Autodesk Inventor part; units mm, degrees
ref_plane "Start plane" through (0, 0, 25) normal (0, 0, 1) x (1, 0, 0)
ref_plane "End plane" through (0, 0, 285) normal (0, 0, 1) x (1, 0, 0)
ref_plane "Work Plane4" through (-8.5, 27.5, 25) normal (0, 0, -1) x (-1, 0, 0)
ref_plane "Start plane" through (0, 0, 25) normal (0, 0, 1) x (1, 0, 0)
ref_plane "End plane" through (0, 0, 285) normal (0, 0, 1) x (1, 0, 0)
sketch "Sketch" plane through (0, 0, 0) normal (0, 0, 1) x (1, 0, 0)
  line L0 (-12.5, -8.5) -> (-12.5, 8.5)
  line L1 (-8.5, 12.5) -> (8.5, 12.5)
  line L2 (12.5, 8.5) -> (12.5, -8.5)
  line L3 (8.5, -12.5) -> (-8.5, -12.5)
  arc A0 (-12.5, -8.5) -> (-8.5, -12.5) centre (-8.5, -8.5) ccw
  arc A1 (12.5, 8.5) -> (8.5, 12.5) centre (8.5, 8.5) ccw
  arc A2 (-8.5, 12.5) -> (-12.5, 8.5) centre (-8.5, 8.5) ccw
  arc A3 (8.5, -12.5) -> (12.5, -8.5) centre (8.5, -8.5) ccw
  arc A4 (-8.5, 10.5) -> (-10.5, 8.5) centre (-8.5, 8.5) ccw
  line L4 (-8.5, 10.5) -> (8.5, 10.5)
  arc A5 (10.5, 8.5) -> (8.5, 10.5) centre (8.5, 8.5) ccw
  line L5 (10.5, 8.5) -> (10.5, -8.5)
  arc A6 (8.5, -10.5) -> (10.5, -8.5) centre (8.5, -8.5) ccw
  line L6 (8.5, -10.5) -> (-8.5, -10.5)
  arc A7 (-10.5, -8.5) -> (-8.5, -10.5) centre (-8.5, -8.5) ccw
  line L7 (-10.5, -8.5) -> (-10.5, 8.5)
  line L8 (0, 18.6598) -> (0, -18.6598) construction
  line L9 (-18.6598, 0) -> (18.6598, 0) construction
  dimension "d7" = 4
  dimension "d9" = 25
  dimension "d11" = 25
  dimension "d12" = 2
  dimension "d15" = 12.5
  dimension "d16" = 12.5
extrude "Body" add sketch "Sketch" along normal up to surface (260 mm away) from surface at 25
sketch "Sketch3" plane through (0, 0, 0) normal (0, 0, 1) x (1, 0, 0)
  line L0 (0, 0) -> (10, 0)
ref_plane "Work Plane3" through (0, 0, 0) normal (0, -1, 0) x (1, 0, 0)
sketch "Sketch4" plane through (0, 0, 0) normal (0, -1, 0) x (1, 0, 0)
  line L0 (-2, 25) -> (12, 25)
  line L1 (-2, 285) -> (12, 285)
  dimension "d18" = 260
ref_plane "Work Plane4" through (-8.5, 27.5, 25) normal (0, 0, -1) x (-1, 0, 0)
split "Split1" plane through (-8.5, 27.5, 25) removes the side toward (0, 0, -1)
ref_plane "Work Plane5" through (8.5, 27.5, 285) normal (0, 0, 1) x (1, 0, 0)
split "Split2" plane through (8.5, 27.5, 285) removes the side toward (0, 0, 1)
equation "\"d7\" = G_IR"
equation "\"d9\" = G_W"
equation "\"d11\" = G_H"
equation "\"d12\" = G_T"
equation "\"d15\" = 0.5 * d9"
equation "\"d16\" = 0.5 * d11"
equation "\"d3\" = G_L"
equation "\"G_W\" = 25"
equation "\"G_H\" = 25"
equation "\"G_T\" = 2"
equation "\"G_IR\" = 4"
equation "\"G_L\" = d18"
equation "\"G_OFFSET_START\" = -25"
equation "\"G_OFFSET_END\" = -25"
equation "\"d13\" = -G_OFFSET_START"
equation "\"d14\" = G_OFFSET_END + B_L"
properties part number "ISO 4019 - 25x25x2 - 260" material "Steel, Mild"
Work out the finished part from the listing and answer in its coordinate system (mm). A direction names the side the tool comes from. Round coordinates to 2 decimals unless told otherwise and drop trailing zeros. Write each loop counter-clockwise with the first axis right and the second up, starting at its lowest first coordinate (ties: lowest second). Pieces come first, ordered by that corner, then holes. Notation, with made-up numbers: M 86,-36.5 L 109,-36.5 A29 cw 109,-6.5 Z; hole C 45.25,1.25 d1. An arc over 180 degrees is marked long. Use a Markdown table: item, result.
1) The part is cut by section C-C on z = 219.5. Give the vertices of the cut face in (x, y).
Taken from the geometry:
| item | result |
|---|---|
| outline | M -12.5,-8.5 A4 ccw -8.5,-12.5 L 8.5,-12.5 A4 ccw 12.5,-8.5 L 12.5,8.5 A4 ccw 8.5,12.5 L -8.5,12.5 A4 ccw -12.5,8.5 Z; hole M -10.5,-8.5 A2 ccw -8.5,-10.5 L 8.5,-10.5 A2 ccw 10.5,-8.5 L 10.5,8.5 A2 ccw 8.5,10.5 L -8.5,10.5 A2 ccw -10.5,8.5 Z |
2) Which of the six approach directions +Z, -Z, +X, -X, +Y, -Y give full straight-line access (tool end or side, diameter ignored) to faces 5 (the face through (0, -10.5, 153)), 6 (the face through (-11, 0, 25))?
Taken from the geometry:
| item | result |
|---|---|
| face 5 | +Z, -Z |
| face 6 | -Z, +X, -X, +Y, -Y |
3) Determine the mould class of faces 1 (the face through (11.297, 11.359, 153.18)), 2 (the face through (0, -12.5, 153)), 3 (the face through (-10.5, 0, 153)), 4 (the face through (-12.5, 0, 153)) for opening direction X: pulls with the +X half, pulls with the -X half, needs draft (parallel to the pull), parting line crosses it, or undercut.
Taken from the geometry:
| item | result |
|---|---|
| face 1 | pulls with the +X half |
| face 2 | needs draft |
| face 3 | undercut |
| face 4 | pulls with the -X half |
4) Consider line 1 (X direction, y = 5, z = 160); line 2 (X direction, y = -10.25, z = 60.5). Determine where each line is inside the solid, lowest interval first. Write a range as [from, to].
Taken from the geometry:
| item | result |
|---|---|
| line 1 | x = [-12.5, -10.5], [10.5, 12.5] |
| line 2 | x = [-12.1, -9.47], [9.47, 12.1] |
5) The part is cut by section A-A on x = -4.75. Give the vertices of the cut face in (y, z).
Taken from the geometry:
| item | result |
|---|---|
| outline | M -12.5,25 L -10.5,25 L -10.5,285 L -12.5,285 Z; M 10.5,25 L 12.5,25 L 12.5,285 L 10.5,285 Z |
